Read the model definition and answer for the solid it produces. Units are mm, in the model's axes. Give positions to 0.01 mm unless a question says otherwise; leave off trailing zeros. Order: outer loops, then holes, each group sorted by start corner. A loop starts at its lowest first (then second) coordinate and runs counter-clockwise, first axis right, second up. Notation, with made-up numbers: M -23,60.25 L 23,60.25 A14 cw 23,81.25 Z; hole C 74,-9 d4. An arc over 180 degrees is marked long. One line per item, written item: value. Start each with the question number.
from build123d import *

# Parameters (mm, degrees)
SKETCH_1_R               = 20
EXTRUDE_1_DEPTH          = 2
SKETCH_2_R               = 1
CUT_EXTRUDE_1_DEPTH      = 2
PATTERN_CIRCULAR_1_COUNT = 3
SKETCH_3_R               = 4
CUT_EXTRUDE_2_DEPTH      = 2


with BuildPart() as part:
    # 草图1 → 凸台-拉伸1 (new body)
    with BuildSketch(Plane.XY):
        Circle(SKETCH_1_R)
    extrude(amount=EXTRUDE_1_DEPTH)

    # 草图2 → 切除-拉伸1 (cut)
    with BuildSketch(Plane.XY.offset(2)):
        with Locations((0, 14)):
            Circle(SKETCH_2_R)
    cut_extrude_1 = extrude(amount=-CUT_EXTRUDE_1_DEPTH, mode=Mode.SUBTRACT)

    # 阵列(圆周)1: 切除-拉伸1 ×3 about axis
    pattern_circular_1_axis = Axis((0, 0, 0), (0, 0, 1))
    for i in range(1, PATTERN_CIRCULAR_1_COUNT):
        add(cut_extrude_1.rotate(pattern_circular_1_axis, i * 360 / PATTERN_CIRCULAR_1_COUNT), mode=Mode.SUBTRACT)

    # 草图3 → 切除-拉伸2 (cut)
    with BuildSketch(Plane.XY.offset(2)):
        Circle(SKETCH_3_R)
    extrude(amount=-CUT_EXTRUDE_2_DEPTH, mode=Mode.SUBTRACT)


solid = part.part
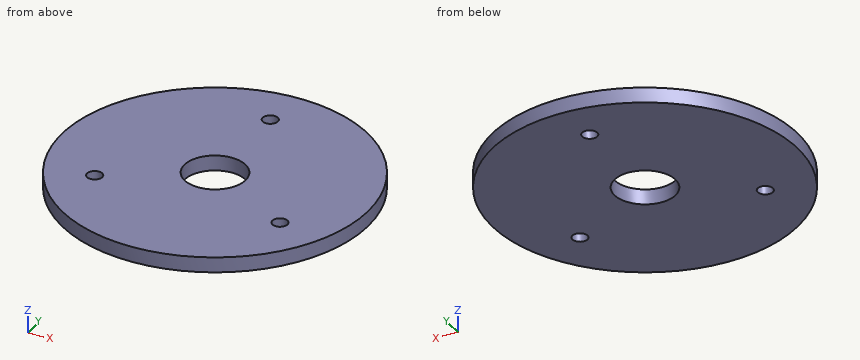
Q1. Find section C-C, the plane y = -7. Give the vertices of the cut face in (x, z) (3 decimals).
Q2. Find section B-B, the plane y = 0. Give the vertices of the cut face in (x, z).
Q3. This flat-tipped pin is pushed along its axis until it touches: pin 1 (1.2 mm diameter, centred on x = -12.12, y = -7, fed in from -Z). Where does it stop, or does it pass through?
Q4. Consider probe 1 along Y at (x, z) = (0, 1.2); probe 2 along Y at (x, z) = (-11, 0.8); probe 3 along X at (y, z) = (-11.5, 1.1). Determine where each line is inside the solid, lowest interval first.
Q5. Find section D-D, the plane z = 0.4. Give the vertices of the cut face in (x, y).
Q6. Find section A-A, the plane x = 0. Give the vertices of the cut face in (y, z), then the cut area to 3 significant figures.
Evaluation:
1. outline: M -18.735,0 L -13.124,0 L -13.124,2 L -18.735,2 Z; M -11.124,0 L 11.124,0 L 11.124,2 L -11.124,2 Z; M 13.124,0 L 18.735,0 L 18.735,2 L 13.124,2 Z
2. outline: M -20,0 L -4,0 L -4,2 L -20,2 Z; M 4,0 L 20,0 L 20,2 L 4,2 Z
3. pin 1: through
4. probe 1: -20 to -4, 4 to 13, 15 to 20
4. probe 2: -16.7 to 16.7
4. probe 3: -16.36 to 16.36
5. outline: C 0,0 d40; hole C -12.12,-7 d2; hole C 0,0 d8; hole C 0,14 d2; hole C 12.12,-7 d2
6. outline: M -20,0 L -4,0 L -4,2 L -20,2 Z; M 4,0 L 13,0 L 13,2 L 4,2 Z; M 15,0 L 20,0 L 20,2 L 15,2 Z
6. area: 60.0 mm2
